Here's the drawing with two shaded views (mm, measured from the low corner). I have some questions. A direction names the side the tool comes from. Give positions to 0.01 mm unless a question says otherwise; leave off trailing zeros. Use one line per item in the form item = value.
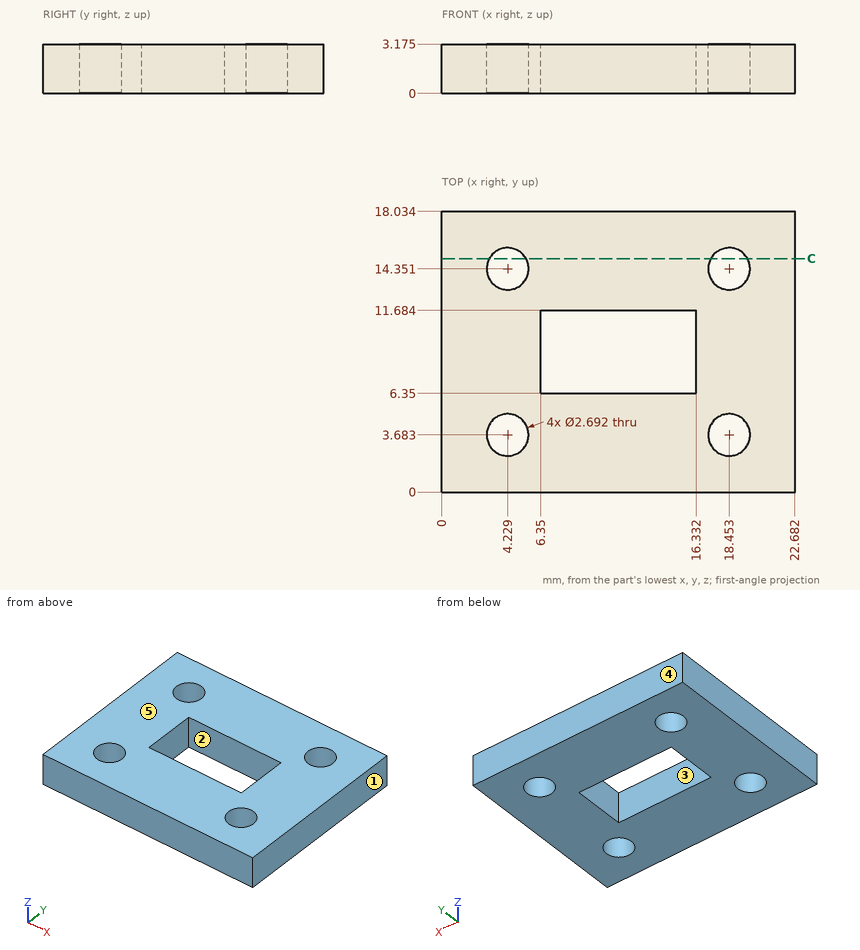
1) I want a section at C-C, the plane y = 15. Count the separate pieces of the cut face and the enclosed holes in it.
Checked values:
separate_pieces = 3
enclosed_holes = 0
2) For pin 1 Ø2.5 at (x, y) = (18.45, 3.68) entering from -Z, with a flat end and sliding along its axis, tell me the tip position at first contact or that it passes through.
Checked values:
pin_1 = through
3) For the marked faces 1 and 2, which set-ups out of +Z, -Z, +X, -X, +Y, -Y let a thin tool reach every point of the face, with its end or its side?
Checked values:
face_1 = +Z, -Z, +X, +Y, -Y
face_2 = +Z, -Z
4) If I drill on L1, parallel to X at y = 8, z = 1.2; L2, parallel to X at y = 14.25, z = 1.1 (1 decimal); L3, parallel to Y at x = 8.75, z = 3.05, over which ranges is the centre line in solid material (lowest first)?
Checked values:
L1 = 0 to 6.35, 16.33 to 22.68
L2 = 0 to 2.9, 5.6 to 17.1, 19.8 to 22.7
L3 = 0 to 6.35, 11.68 to 18.03
5) Thinking about a two-plate mould opening in Y: for the marked faces 3, 4 and 5, which applies, released by +Y, released by -Y, zero draft, split by the parting line, or undercut?
Checked values:
face_3 = undercut
face_4 = released by +Y
face_5 = zero draft
